Solid Edge part; units mm, degrees
sketch "Sketch1" plane through (0, 0, 0) normal (0, 0, 1) x (1, 0, 0)
  line L0 (15, 19) -> (-15, 19)
  arc A0 (-15, 19) -> (-19, 15) centre (-15, 15) ccw
  line L1 (-19, 15) -> (-19, -15)
  arc A1 (-19, -15) -> (-15, -19) centre (-15, -15) ccw
  line L2 (-15, -19) -> (15, -19)
  arc A2 (15, -19) -> (19, -15) centre (15, -15) ccw
  line L3 (19, -15) -> (19, 15)
  arc A3 (15, 19) -> (19, 15) centre (15, 15) cw
extrude "Protrusion1" add sketch "Sketch1" along normal blind 4
sketch "Sketch2" plane through (0, 0, 0) normal (0, 0, -1) x (-1, 0, 0)
  circle A0 centre (0, 0) radius 16
extrude "Protrusion2" add sketch "Sketch2" along normal blind 3
sketch "Sketch3" plane through (0, 0, -3) normal (0, 0, -1) x (-1, 0, 0)
  circle A0 centre (0, 0) radius 10
extrude "Protrusion3" add sketch "Sketch3" along normal blind 14.8
sketch "Sketch4" plane through (0, 0, 4) normal (0, 0, 1) x (1, 0, 0)
  circle A0 centre (0, 0) radius 12
extrude "Cutout1" cut sketch "Sketch4" against normal blind 5
sketch "Sketch5" plane through (0, 0, -1) normal (0, 0, 1) x (1, 0, 0)
  circle A0 centre (0, 0) radius 6.55
extrude "Cutout2" cut sketch "Sketch5" against normal up to next
hole "Hole1" at (-14.5, 14.5, 4) direction (0, 0, -1) diameter 4 end up to next
hole "Hole2" at (14.5, 14.5, 4) direction (0, 0, -1) diameter 4 end up to next
hole "Hole3" at (14.5, -14.5, 4) direction (0, 0, -1) diameter 4 end up to next
hole "Hole4" at (-14.5, -14.5, 4) direction (0, 0, -1) diameter 4 end up to next
properties part number "PLATE1" material "410 Stainless Steel"
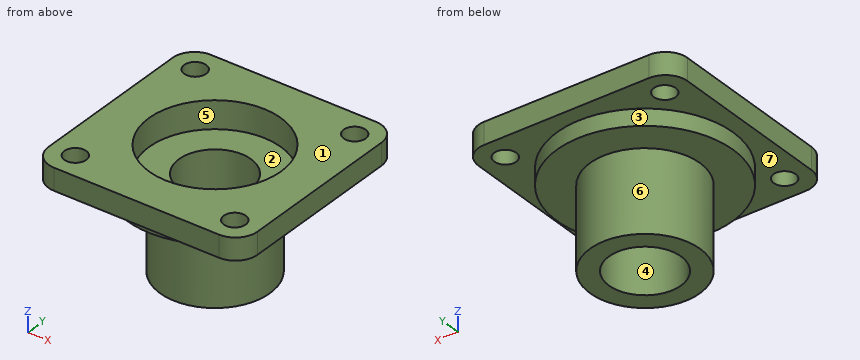
The model under review builds one solid part; all positions refer to its coordinate system, in mm. Face numbers are marked on the shaded views. A direction names the side the tool comes from. Give positions to 0.01 mm unless a question says otherwise; leave off trailing zeros. Write each loop counter-clockwise with the first axis right and the second up, starting at its lowest first coordinate (ties: lowest second). Pieces come first, ordered by that corner, then holes. Notation, with made-up numbers: M -2,-31 L 7,-31 A22 ccw 7,-24 Z; hole C -40,-12.75 d9. An arc over 180 degrees is marked long. Write item = value, one per line. Start each with the question number.
Q1. Machinability: for the marked faces 1, 2 and 3, which of the approach directions +Z, -Z, +X, -X, +Y, -Y give a long, thin tool a straight path to every point of the face, cutting with its end or side? Answer none if there is none.
Q2. We need section C-C (x = -14.5). State the section outline as (y, z) points.
Q3. We need section A-A (z = 0.5). State the section outline as (x, y) points.
Q4. We need section B-B (y = 0). State the section outline as (x, z) points, plus the area to 3 significant figures.
Q5. Mouldability with a two-part tool opening along Y and no side actions: class the marked faces 4, 5, 6 and 7 as released by +Y, released by -Y, zero draft, split by the parting line, or undercut.
Q6. For line 1 (X direction, y = -14.5, z = 1.2); line 2 (Y direction, x = 0, z = 0.9), list the stretches that pass through material, from the lowest coordinate up.
Q7. Clearance check with flat-ended pins moving along their axes: pin 1 (7 mm diameter, centred on x = -1.5, y = -5.5, fed in from +Z); pin 2 (12 mm diameter, centred on x = -1, z = -10.5, fed in from +Y); pin 3 (12 mm diameter, centred on y = -2, z = -9.5, fed in from -X). State where each tip first meets the part, or that it passes through.
Result set:
q1.face_1 = +Z, +X, -X, +Y, -Y
q1.face_2 = +Z
q1.face_3 = -Z
q2.outline = M -19,0 L -16.5,0 L -16.5,4 L -19,4 Z; M -12.5,0 L -6.76,0 L -6.76,-3 L 6.76,-3 L 6.76,0 L 12.5,0 L 12.5,4 L -12.5,4 Z; M 16.5,0 L 19,0 L 19,4 L 16.5,4 Z
q3.outline = M -19,-15 A4 ccw -15,-19 L 15,-19 A4 ccw 19,-15 L 19,15 A4 ccw 15,19 L -15,19 A4 ccw -19,15 Z; hole C -14.5,-14.5 d4; hole C -14.5,14.5 d4; hole C 0,0 d24; hole C 14.5,-14.5 d4; hole C 14.5,14.5 d4
q4.outline = M -19,0 L -16,0 L -16,-3 L -10,-3 L -10,-17.8 L -6.55,-17.8 L -6.55,-1 L -12,-1 L -12,4 L -19,4 Z; M 6.55,-17.8 L 10,-17.8 L 10,-3 L 16,-3 L 16,0 L 19,0 L 19,4 L 12,4 L 12,-1 L 6.55,-1 Z
q4.area = 204 mm2
q5.face_4 = undercut
q5.face_5 = undercut
q5.face_6 = split by the parting line
q5.face_7 = zero draft
q6.line_1 = -19 to -16.5, -12.5 to 12.5, 16.5 to 19
q6.line_2 = -19 to -12, 12 to 19
q7.pin_1 = -1
q7.pin_2 = 10
q7.pin_3 = -10
